from build123d import *

# Parameters (mm, degrees)
SKETCH1_R      = 1.27635
EXTRUDE1_DEPTH = 25.4


with BuildPart() as part:
    # Sketch1 → Extrude1 (new body)
    with BuildSketch(Plane.XY):
        with BuildLine():
            Line((-2.266074779, 2.792259021), (-3.597719195, 4.250869712))
            ThreePointArc((-3.597719195, 4.250869712), (-3.707979565, 4.804147382), (-3.239236773, 5.118080056))
            Line((-3.239236773, 5.118080056), (-2.12725, 5.1181))
            ThreePointArc((-2.12725, 5.1181), (-1.768039755, 5.266889755), (-1.61925, 5.6261))
            Line((-1.61925, 5.6261), (-1.61925, 5.731127227))
            ThreePointArc((-1.61925, 5.731127227), (-1.762294622, 6.084500719), (-2.110872134, 6.238864921))
            Line((-2.110872134, 6.238864921), (-5.55625, 6.3499873))
            ThreePointArc((-5.55625, 6.3499873), (-6.117516008, 6.117503308), (-6.35, 5.5562373))
            Line((-6.35, 5.5562373), (-6.35, -5.55625))
            ThreePointArc((-6.35, -5.55625), (-6.117516008, -6.117516008), (-5.55625, -6.35))
            Line((-5.55625, -6.35), (5.55625, -6.35))
            ThreePointArc((5.55625, -6.35), (6.117516008, -6.117516008), (6.35, -5.55625))
            Line((6.35, -5.55625), (6.2388496, -2.110867))
            ThreePointArc((6.2388496, -2.110867), (6.084481448, -1.762300959), (5.73111497, -1.6192627))
            Line((5.73111497, -1.6192627), (5.6261, -1.6192627))
            ThreePointArc((5.6261, -1.6192627), (5.266889755, -1.768052455), (5.1181, -2.1272627))
            Line((5.1181, -2.1272627), (5.118086781, -3.239226147))
            ThreePointArc((5.118086781, -3.239226147), (4.804155079, -3.707969591), (4.250877181, -3.59771037))
            Line((4.250877181, -3.59771037), (2.7922601, -2.2660864))
            ThreePointArc((2.7922601, -2.2660864), (2.351781222, -1.606857234), (2.1971, -0.8292465))
            Line((2.1971, -0.8292465), (2.1971, 0.8292338))
            ThreePointArc((2.1971, 0.8292338), (2.35177885, 1.606851508), (2.792259021, 2.266087479))
            Line((2.792259021, 2.266087479), (4.250877574, 3.596983984))
            ThreePointArc((4.250877574, 3.596983984), (4.804155516, 3.707243364), (5.1180873, 3.238499886))
            Line((5.1180873, 3.238499886), (5.1181, 2.12725))
            ThreePointArc((5.1181, 2.12725), (5.266889755, 1.768039755), (5.6261, 1.61925))
            Line((5.6261, 1.61925), (5.731114527, 1.61925))
            ThreePointArc((5.731114527, 1.61925), (6.084488115, 1.762294714), (6.23885223, 2.1108724))
            Line((6.23885223, 2.1108724), (6.35, 5.55625))
            ThreePointArc((6.35, 5.55625), (6.117516008, 6.117516008), (5.55625, 6.35))
            Line((5.55625, 6.35), (2.110872134, 6.238864921))
            ThreePointArc((2.110872134, 6.238864921), (1.762294622, 6.084500719), (1.61925, 5.731127227))
            Line((1.61925, 5.731127227), (1.61925, 5.6261))
            ThreePointArc((1.61925, 5.6261), (1.768039755, 5.266889755), (2.12725, 5.1181))
            Line((2.12725, 5.1181), (3.238489261, 5.118094023))
            ThreePointArc((3.238489261, 5.118094023), (3.70723339, 4.804163213), (3.596975159, 4.250885042))
            Line((3.596975159, 4.250885042), (2.266081683, 2.792263725))
            ThreePointArc((2.266081683, 2.792263725), (1.606847146, 2.351789743), (0.8292338, 2.1971127))
            Line((0.8292338, 2.1971127), (-0.8292338, 2.1971))
            ThreePointArc((-0.8292338, 2.1971), (-1.606846535, 2.35177679), (-2.266074779, 2.792259021))
        make_face()
        Circle(SKETCH1_R, mode=Mode.SUBTRACT)
        with BuildLine():
            Line((-5.1180873, -3.238499886), (-5.118086781, 3.239226147))
            ThreePointArc((-5.118086781, 3.239226147), (-4.804155079, 3.707969591), (-4.250877181, 3.59771037))
            Line((-4.250877181, 3.59771037), (-2.792246321, 2.266087479))
            ThreePointArc((-2.792246321, 2.266087479), (-2.35176409, 1.606859235), (-2.1970873, 0.8292465))
            Line((-2.1970873, 0.8292465), (-2.1971, -0.8292465))
            ThreePointArc((-2.1971, -0.8292465), (-2.35177679, -1.606859235), (-2.792259021, -2.266087479))
            Line((-2.792259021, -2.266087479), (-4.250877574, -3.596983984))
            ThreePointArc((-4.250877574, -3.596983984), (-4.804155516, -3.707243364), (-5.1180873, -3.238499886))
        make_face(mode=Mode.SUBTRACT)
        with BuildLine():
            Line((0.8292465, -2.1970873), (-0.8292465, -2.1971))
            ThreePointArc((-0.8292465, -2.1971), (-1.606859235, -2.35177679), (-2.266087479, -2.792259021))
            Line((-2.266087479, -2.792259021), (-3.596983984, -4.250877574))
            ThreePointArc((-3.596983984, -4.250877574), (-3.707243364, -4.804155516), (-3.238499886, -5.1180873))
            Line((-3.238499886, -5.1180873), (3.239226147, -5.118086781))
            ThreePointArc((3.239226147, -5.118086781), (3.707969591, -4.804155079), (3.59771037, -4.250877181))
            Line((3.59771037, -4.250877181), (2.266087479, -2.792246321))
            ThreePointArc((2.266087479, -2.792246321), (1.606859235, -2.35176409), (0.8292465, -2.1970873))
        make_face(mode=Mode.SUBTRACT)
    extrude(amount=EXTRUDE1_DEPTH)


solid = part.part
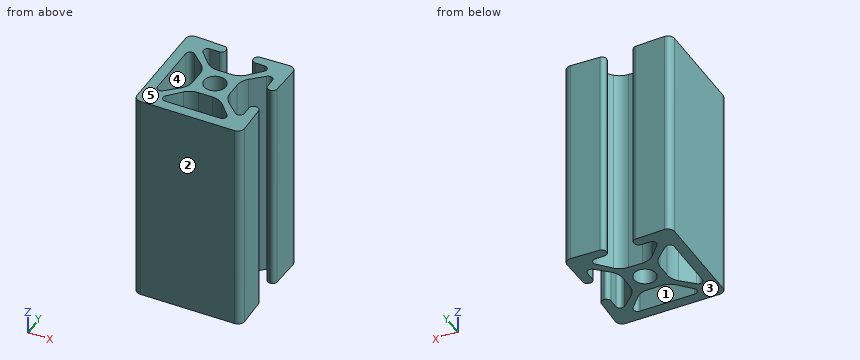
CAD build for the part. Positions are in the model's coordinates, mm. Face numbers are marked on the shaded views. A direction names the side the tool comes from. Give positions to 0.01 mm unless a question says otherwise; leave off trailing zeros. Write each loop counter-clockwise with the first axis right and the second up, starting at its lowest first coordinate (ties: lowest second). Pieces come first, ordered by that corner, then holes. Notation, with made-up numbers: M 35.5,14 L 84.5,14 A32 ccw 84.5,45 Z; hole C -34,60 d11. An arc over 180 degrees is marked long. Put each result on its own line as item: value. Start each with the question number.
(1) Mould opens along Y. For the marked faces 1, 2 and 3 say: +Y half, -Y half, draft (parallel to the pull), parting line (faces both ways), or undercut.
(2) Probe L1, parallel to Y at x = 0, z = 7; L2, parallel to Y at x = 2.75, z = 23.5; L3, parallel to X at y = -3.5, z = 20.5. List the from-to ranges inside material, lowest first.
(3) Band-saw the part on C-C, the plane z = 3.75. Give the number of separate pieces and of enclosed holes in the cut face, and give its area (3 significant figures).
(4) Which spindle directions (+Z, -Z, +X, -X, +Y, -Y) get a long thin tool onto all of the face, cutting with end or side? Do the marked faces 4 and 5. Say none if no direction does.
(5) Band-saw the part on A-A, the plane y = 0. Write the cut outline in (x, z).
(6) Band-saw the part on D-D, the plane x = 4. Write the cut outline in (y, z).
(7) Flat gauge pins, fed straight in: pin 1 Ø5 at (x, y) = (-4, -1) entering from -Z; pin 2 Ø0.8 at (y, z) = (-0.5, 12.5) entering from +X; pin 3 Ø5 at (x, z) = (1, 9.5) entering from +Y; pin 4 Ø0.8 at (x, z) = (0, 13.5) entering from +Y. Where does each tip first touch, or does it go through?
Response values:
1. face 1: undercut
1. face 2: -Y half
1. face 3: draft
2. L1: y = -6.35 to -5.12, -2.2 to -1.28, 1.28 to 2.2
2. L2: y = -6.35 to -5.12, -3.32 to -2.22, 2.22 to 3.32, 5.12 to 6.26
2. L3: x = -6.35 to -5.05, -4.14 to -2.91, 2.91 to 4.14, 5.05 to 6.28
3. separate pieces: 1
3. enclosed holes: 3
3. area: 77.9 mm2
4. face 4: +Z, -Z
4. face 5: +Z, +X, -X, +Y, -Y
5. outline: M -6.35,0 L -5.12,0 L -5.12,25.4 L -6.35,25.4 Z; M -2.2,0 L -1.28,0 L -1.28,25.4 L -2.2,25.4 Z; M 1.28,0 L 2.2,0 L 2.2,25.4 L 1.28,25.4 Z
6. outline: M -6.35,0 L -3.37,0 L -3.37,25.4 L -6.35,25.4 Z; M 3.37,0 L 6.3,0 L 6.3,25.4 L 3.37,25.4 Z
7. pin 1: stops at z = 0
7. pin 2: stops at x = 2.2
7. pin 3: stops at y = 6.28
7. pin 4: stops at y = 2.2
